For this review, take the finished solid that the model builds, in its own axes (mm). Face numbers are marked on the shaded views. A direction names the side the tool comes from. Give positions to 0.01 mm unless a question says otherwise; leave off trailing zeros. Order: outer loops, then holes, each group sorted by start corner. A loop starts at its lowest first (then second) coordinate and runs counter-clockwise, first axis right, second up. Notation, with made-up numbers: (50, -35) - (90, -35) arc R26 cw to (90, -11) - close; hole circle Ø7 at (12.5, -23.75). An arc over 180 degrees is marked (long way). One line per item, written item: value.
```python
from build123d import *
from OCP.BRepFilletAPI import BRepFilletAPI_MakeChamfer

# Parameters (mm, degrees)
SKETCH1_W           = 70
SKETCH1_H           = 100
BOSS_EXTRUDE1_DEPTH = 16.5
CUT_EXTRUDE1_DEPTH  = 12
BOSS_EXTRUDE2_DEPTH = 4
BOSS_EXTRUDE3_DEPTH = 4
CHAMFER1_SIZE       = 4
CHAMFER1_SIZE2      = 4.335908163


with BuildPart() as part:
    # Sketch1 → Boss-Extrude1 (new, symmetric)
    with BuildSketch(Plane.XY):
        with Locations((35, 50)):
            Rectangle(SKETCH1_W, SKETCH1_H)
    extrude(amount=BOSS_EXTRUDE1_DEPTH, both=True)

    # Sketch2 → Cut-Extrude1 (cut, symmetric)
    with BuildSketch(Plane.XY):
        Polygon((5, 100), (65, 100), (57.511201523, 0), (12.488798477, 0), align=None)
    extrude(amount=CUT_EXTRUDE1_DEPTH, both=True, mode=Mode.SUBTRACT)

    # Sketch3 → Boss-Extrude2 (add)
    with BuildSketch(Plane.XZ):
        Polygon((0, 16.5), (20, 31.5), (50, 31.5), (70, 16.5), align=None)
        Polygon((50, -31.5), (70, -16.5), (0, -16.5), (20, -31.5), align=None)
    extrude(amount=-BOSS_EXTRUDE2_DEPTH)

    # Sketch5 → Boss-Extrude3 (add, symmetric)
    with BuildSketch(Plane.ZY.offset(-35)):
        Polygon((-16.5, 100), (-31.5, 4), (-16.5, 4), align=None)
        Polygon((31.5, 4), (16.5, 4), (16.5, 100), align=None)
    extrude(amount=BOSS_EXTRUDE3_DEPTH, both=True)

    # Chamfer1: one chamfer whose edges measure the first distance from different faces: ONE call of the kernel's chamfer builder (chamfer() names one face for all edges)
    chamfer1_edges_1 = [part.edges().sort_by_distance(p)[0] for p in [
        (35, 100, -12),
        (35, 100, 12),
    ]]
    chamfer1_edges_2 = [part.edges().sort_by_distance(p)[0] for p in [
        (5, 100, 0),
    ]]
    chamfer1_side_2 = [part.faces().sort_by_distance(p)[0] for p in [
        (69.226113703, 100, 0),
    ]]
    chamfer1_edges_3 = [part.edges().sort_by_distance(p)[0] for p in [
        (65, 100, 0),
    ]]
    chamfer1_side_3 = [part.faces().sort_by_distance(p)[0] for p in [
        (61.255600762, 50, 0),
    ]]
    chamfer1 = BRepFilletAPI_MakeChamfer(part.part.solid().wrapped)
    for e in chamfer1_edges_1:
        chamfer1.Add(CHAMFER1_SIZE, e.wrapped)
    for e in chamfer1_edges_2:
        chamfer1.Add(CHAMFER1_SIZE, CHAMFER1_SIZE2, e.wrapped, chamfer1_side_2[0].wrapped)  # the first distance lies on this face
    for e in chamfer1_edges_3:
        chamfer1.Add(CHAMFER1_SIZE, CHAMFER1_SIZE2, e.wrapped, chamfer1_side_3[0].wrapped)  # the first distance lies on this face
    add(Compound.cast(chamfer1.Shape()), mode=Mode.REPLACE)


solid = part.part
```
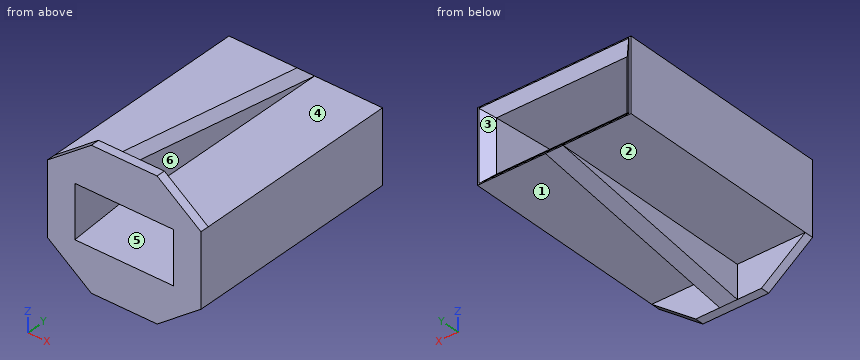
(1) Take a section at C-C (y = 17.5). Write out the cut boundary in (x, z).
Answers below:
outline: (0, -16.5) - (31, -16.5) - (31, -29.39) - (39, -29.39) - (39, -16.5) - (70, -16.5) - (70, 16.5) - (39, 16.5) - (39, 29.39) - (31, 29.39) - (31, 16.5) - (0, 16.5) - close; hole (11.18, -12) - (58.82, -12) - (58.82, 12) - (11.18, 12) - close
(2) Take a section at A-A (x = 56). Write out the cut boundary in (y, z).
Answers below:
outline: (0, -27) - (4, -27) - (4, -16.5) - (100, -16.5) - (100, -16) - (96, -12) - (0, -12) - close; (0, 12) - (96, 12) - (100, 16) - (100, 16.5) - (4, 16.5) - (4, 27) - (0, 27) - close
(3) For P1, Ø7.5, axis at y = 44, z = -24, coming from the +X side; P2, Ø12, axis at x = 18.5, z = 23, coming from the -Y side; P3, Ø12, axis at x = 14, z = -23, coming from the +Y side; P4, Ø15.5, axis at x = 60.5, y = 43, coming from the -Z side, all flat-tipped, find the tip position at first contact; note any pin that passes through.
Answers below:
P1: stops at x = 39
P2: stops at y = 0
P3: stops at y = 4
P4: stops at z = -16.5
(4) Take a section at D-D (z = 21). Write out the cut boundary in (x, y).
Answers below:
outline: (6, 0) - (64, 0) - (64, 4) - (39, 4) - (39, 71.2) - (31, 71.2) - (31, 4) - (6, 4) - close
(5) Wall thickness on line 1 (Z direction, x = 57, y = 24); line 2 (X direction, y = 91, z = -9); line 3 (Z direction, x = 67.5, y = 25.5): over which ranges is each line inside the solid? List them lowest first. Write a range as from..to.
Answers below:
line 1: z = -16.5..-12, 12..16.5
line 2: x = 0..5.67, 64.33..70
line 3: z = -16.5..16.5
(6) Machinability: for the marked faces 1, 2 and 3, which of the approach directions +Z, -Z, +X, -X, +Y, -Y give a long, thin tool a straight path to every point of the face, cutting with its end or side? Answer none if there is none.
Answers below:
face 1: -Z, +X, +Y
face 2: -Z, -X, +Y
face 3: +Y
(7) Take a section at B-B (z = 1). Write out the cut boundary in (x, y).
Answers below:
outline: (0, 0) - (12.49, 0) - (5.32, 95.68) - (1, 100) - (0, 100) - close; (57.51, 0) - (70, 0) - (70, 100) - (69.34, 100) - (64.7, 96.01) - close
(8) Draft analysis for pull direction X (two halves, no side actions). For the marked faces 4, 5 and 6, state which applies: pulls with the +X half, pulls with the -X half, needs draft (parallel to the pull), parting line crosses it, or undercut.
Answers below:
face 4: needs draft
face 5: undercut
face 6: pulls with the +X half
